```python
from build123d import *

# Parameters (mm, degrees)
PAD_DEPTH = 2.5


with BuildPart() as part:
    # Sketch → Pad (new body, symmetric)
    with BuildSketch(Plane.YZ):
        with BuildLine():
            Line((10, -2.55), (10, 2.55))
            Line((10, 2.55), (0, 2.55))
            Line((0, 2.55), (0, 10))
            Line((0, 10), (20, 10))
            ThreePointArc((20, 10), (17.466185, 0), (20, -10))
            Line((20, -10), (0, -10))
            Line((0, -10), (0, -2.55))
            Line((0, -2.55), (10, -2.55))
        make_face()
    extrude(amount=PAD_DEPTH, both=True)


solid = part.part
```
Could you check a few things on this model? Use its own coordinates, in mm. A direction names the side the tool comes from. Coordinates: 2 decimals unless noted, no trailing zeros. Loops run counter-clockwise (first coordinate to the right, second up) from the corner with the lowest first, then second, coordinate; pieces in that order, holes last.
1) Which directions (+Z, -Z, +X, -X, +Y, -Y) give clear straight access to the entire face, cutting with the end or side of a thin tool? Please do faces 1 (the face through (0, 5, -2.55)), 2 (the face through (0, 0, -6)).
Reported:
face 1: +X, -X, -Y
face 2: +Z, -Z, +X, -X, -Y
2) Imagine slicing it at A-A (y = 5). List the corners of the cut face in (x, z) for me.
Reported:
outline: (-2.5, -10) - (2.5, -10) - (2.5, -2.55) - (-2.5, -2.55) - close; (-2.5, 2.55) - (2.5, 2.55) - (2.5, 10) - (-2.5, 10) - close
3) Will this pin go through, and if not, where does the flat tip stop? pin 1 Ø1.5 at (x, z) = (-1, -0.5) entering from -Y.
Reported:
pin 1: stops at y = 10
4) Thinking about a two-plate mould opening in Z: for faces 3 (the face through (0, 10, -10)), 4 (the face through (0, 10, 0)), 5 (the face through (-2.5, 12, 0)), which applies, released by +Z, released by -Z, zero draft, split by the parting line, or undercut?
Reported:
face 3: released by -Z
face 4: undercut
face 5: zero draft
5) Imagine slicing it at B-B (x = 0.4). List the corners of the cut face in (y, z) for me, and give its area (3 significant figures).
Reported:
outline: (0, -10) - (20, -10) arc R21 cw to (20, 10) - (0, 10) - (0, 2.55) - (10, 2.55) - (10, -2.55) - (0, -2.55) - close
area: 315 mm2
6) Please list where these lines run through material, in increasing order: line 1 along Z through (x, y) = (-0.9, 9.25); line 2 along Y through (x, z) = (-2.2, 7.25); line 3 along Y through (x, z) = (-1, -6).
Reported:
line 1: z = -10 to -2.55, 2.55 to 10
line 2: y = 0 to 18.76
line 3: y = 0 to 18.34
7) Imagine slicing it at D-D (z = 0.5). List the corners of the cut face in (x, y) for me, and give its area (3 significant figures).
Reported:
outline: (-2.5, 10) - (2.5, 10) - (2.5, 17.47) - (-2.5, 17.47) - close
area: 37.4 mm2
8) Imagine slicing it at C-C (z = 8.75). List the corners of the cut face in (x, y) for me, and give its area (3 significant figures).
Reported:
outline: (-2.5, 0) - (2.5, 0) - (2.5, 19.38) - (-2.5, 19.38) - close
area: 96.9 mm2
